For this review, take the finished solid that the model builds, in its own axes (mm). Give positions to 0.01 mm unless a question says otherwise; leave off trailing zeros. Loops run counter-clockwise (first coordinate to the right, second up) from the corner with the lowest first, then second, coordinate; pieces in that order, holes last.
```python
from build123d import *

# Parameters (mm, degrees)
SKETCH1_W           = 52.2
SKETCH1_H           = 29.3
BOSS_EXTRUDE1_DEPTH = 9.7
SKETCH2_R           = 1
BOSS_EXTRUDE2_DEPTH = 7
FILLET1_R           = 2
FILLET2_R           = 2
FILLET3_R           = 2
FILLET4_R           = 2


with BuildPart() as part:
    # Sketch1 → Boss-Extrude1 (new body)
    with BuildSketch(Plane.XY):
        Rectangle(SKETCH1_W, SKETCH1_H)
    extrude(amount=BOSS_EXTRUDE1_DEPTH)

    # Sketch2 → Boss-Extrude2 (add)
    with BuildSketch(Plane.ZY.offset(26.1)):
        with Locations(Location((4.7, -13.15, 0), (0, 0, 180))):
            Circle(SKETCH2_R)
        with Locations(Location((4.7, -10.15, 0), (0, 0, 180))):
            Circle(SKETCH2_R)
    extrude(amount=BOSS_EXTRUDE2_DEPTH)

    # Fillet1
    fillet1_edges = [part.edges().sort_by_distance(p)[0] for p in [
        (26.1, 0, 9.7),
        (0, 14.65, 9.7),
        (-26.1, 0, 9.7),
        (0, -14.65, 9.7),
    ]]
    fillet(fillet1_edges, radius=FILLET1_R)

    # Fillet2
    fillet2_edges = [part.edges().sort_by_distance(p)[0] for p in [
        (0, 14.65, 0),
        (26.1, 0, 0),
        (0, -14.65, 0),
        (-26.1, 0, 0),
    ]]
    fillet(fillet2_edges, radius=FILLET2_R)

    # Fillet3
    # the kernel refuses this fillet: 2 mm, written as the material it takes off along each edge
    with BuildSketch(Plane(origin=(-24.1, 12.65, 7.7), x_dir=(0, 1, 0), z_dir=(-1, 0, 0))) as fillet3_piece_1_section:
        Polygon((0, 0), (FILLET3_R, 0), (FILLET3_R, -FILLET3_R), (0, -FILLET3_R), align=None)
    fillet3_piece_1 = extrude(amount=FILLET3_R, mode=Mode.PRIVATE)
    fillet3_piece_1 = fillet3_piece_1 - Plane(origin=(-24.1, 12.65, 7.7), x_dir=(0, -0.7071067811865475, -0.7071067811865475), z_dir=(-1, 0, 0)) * Sphere(FILLET3_R, mode=Mode.PRIVATE)
    add(fillet3_piece_1, mode=Mode.SUBTRACT)
    with BuildSketch(Plane(origin=(-24.1, 12.65, 2), x_dir=(0, 1, 0), z_dir=(-1, 0, 0))) as fillet3_piece_2_section:
        Polygon((0, 0), (FILLET3_R, 0), (FILLET3_R, FILLET3_R), (0, FILLET3_R), align=None)
    fillet3_piece_2 = extrude(amount=FILLET3_R, mode=Mode.PRIVATE)
    fillet3_piece_2 = fillet3_piece_2 - Plane(origin=(-24.1, 12.65, 2), x_dir=(0, -0.7071067811865475, 0.7071067811865475), z_dir=(-1, 0, 0)) * Sphere(FILLET3_R, mode=Mode.PRIVATE)
    add(fillet3_piece_2, mode=Mode.SUBTRACT)
    with BuildSketch(Plane(origin=(-26.1, 14.65, 2), x_dir=(0, -1, 0), z_dir=(0, 0, 1))) as fillet3_piece_3:
        with BuildLine():
            CenterArc((FILLET3_R, FILLET3_R), FILLET3_R, 180, 90)
            Line((0, FILLET3_R), (0, 0))
            Line((0, 0), (FILLET3_R, 0))
        make_face()
    extrude(amount=5.7, mode=Mode.SUBTRACT)

    # Fillet4
    # the kernel refuses this fillet: 2 mm, written as the material it takes off along each edge
    with BuildSketch(Plane(origin=(24.1, -12.65, 7.7), x_dir=(1, 0, 0), z_dir=(0, -1, 0))) as fillet4_piece_1_section:
        Polygon((0, 0), (FILLET4_R, 0), (FILLET4_R, FILLET4_R), (0, FILLET4_R), align=None)
    fillet4_piece_1 = extrude(amount=FILLET4_R, mode=Mode.PRIVATE)
    fillet4_piece_1 = fillet4_piece_1 - Plane(origin=(24.1, -12.65, 7.7), x_dir=(-0.7071067811865475, 0, -0.7071067811865475), z_dir=(0, -1, 0)) * Sphere(FILLET4_R, mode=Mode.PRIVATE)
    add(fillet4_piece_1, mode=Mode.SUBTRACT)
    with BuildSketch(Plane(origin=(24.1, -12.65, 2), x_dir=(1, 0, 0), z_dir=(0, -1, 0))) as fillet4_piece_2_section:
        Polygon((0, 0), (FILLET4_R, 0), (FILLET4_R, -FILLET4_R), (0, -FILLET4_R), align=None)
    fillet4_piece_2 = extrude(amount=FILLET4_R, mode=Mode.PRIVATE)
    fillet4_piece_2 = fillet4_piece_2 - Plane(origin=(24.1, -12.65, 2), x_dir=(-0.7071067811865475, 0, 0.7071067811865475), z_dir=(0, -1, 0)) * Sphere(FILLET4_R, mode=Mode.PRIVATE)
    add(fillet4_piece_2, mode=Mode.SUBTRACT)
    with BuildSketch(Plane(origin=(26.1, -14.65, 2), x_dir=(-1, 0, 0), z_dir=(0, 0, 1))) as fillet4_piece_3:
        with BuildLine():
            CenterArc((FILLET4_R, -FILLET4_R), FILLET4_R, 90, 90)
            Line((0, -FILLET4_R), (0, 0))
            Line((0, 0), (FILLET4_R, 0))
        make_face()
    extrude(amount=5.7, mode=Mode.SUBTRACT)


solid = part.part
```
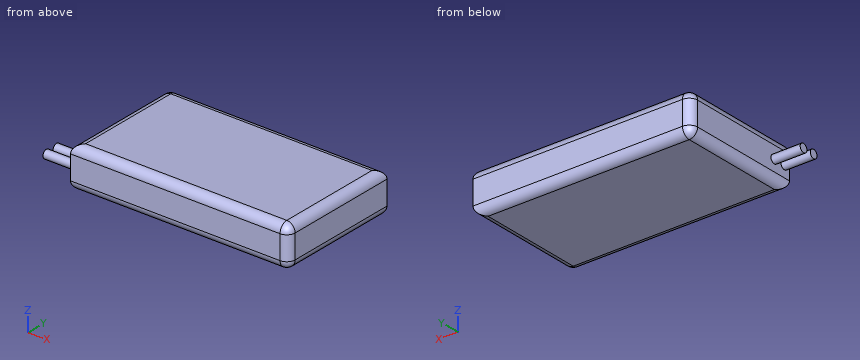
Q1. Consider section B-B on z = 4.7. Give the boundary of the cut face in (x, y), plus the area to 3 significant figures.
Answers:
outline: (-33.1, -14.15) - (-26.1, -14.15) - (-26.1, -14.65) - (24.1, -14.65) arc R2 ccw to (26.1, -12.65) - (26.1, 14.65) - (-24.1, 14.65) arc R2 ccw to (-26.1, 12.65) - (-26.1, -9.15) - (-33.1, -9.15) - (-33.1, -11.15) - (-26.1, -11.15) - (-26.1, -12.15) - (-33.1, -12.15) - close
area: 1,560 mm2
Q2. For probe 1 along X at (y, z) = (-7.75, 3); probe 2 along Z at (x, y) = (-25, -8.75); probe 3 along Y at (x, z) = (-28, 4.25), list the stretches that pass through material, from the lowest coordinate up.
Answers:
probe 1: x = -26.1 to 26.1
probe 2: z = 0.21 to 9.49
probe 3: y = -14.04 to -12.26, -11.04 to -9.26
Q3. Consider section C-C on y = 2. Give the boundary of the cut face in (x, z), plus the area to 3 significant figures.
Answers:
outline: (-26.1, 2) arc R2 ccw to (-24.1, 0) - (24.1, 0) arc R2 ccw to (26.1, 2) - (26.1, 7.7) arc R2 ccw to (24.1, 9.7) - (-24.1, 9.7) arc R2 ccw to (-26.1, 7.7) - close
area: 503 mm2
Q4. For pin 1 Ø3 at (x, z) = (-26, 7) entering from +Y; pin 2 Ø3 at (y, z) = (3, 5) entering from -X, all flat-tipped, find the tip position at first contact; note any pin that passes through.
Answers:
pin 1: stops at y = 14.61
pin 2: stops at x = -26.1
Q5. Consider section A-A on y = -10.15. Give the boundary of the cut face in (x, z).
Answers:
outline: (-33.1, 3.7) - (-26.1, 3.7) - (-26.1, 2) arc R2 ccw to (-24.1, 0) - (24.1, 0) arc R2 ccw to (26.1, 2) - (26.1, 7.7) arc R2 ccw to (24.1, 9.7) - (-24.1, 9.7) arc R2 ccw to (-26.1, 7.7) - (-26.1, 5.7) - (-33.1, 5.7) - close
